CAD build for the part. Positions are in the model's coordinates, mm. A direction names the side the tool comes from. Round coordinates to 2 decimals unless told otherwise and drop trailing zeros. Order: outer loops, then holes, each group sorted by start corner. A loop starts at its lowest first (then second) coordinate and runs counter-clockwise, first axis right, second up. Notation, with made-up numbers: M 34,11 L 55,11 A35 cw 55,44 Z; hole C 60,85 d3. An arc over 180 degrees is marked long. Answer as a JSON object with one key per item and string values.
```python
from build123d import *

# Parameters (mm, degrees)
EXTRUDE_1_DEPTH     = 25
SKETCH_2_R          = 1.7
CUT_EXTRUDE_1_DEPTH = 25
CUT_EXTRUDE_START   = -7.5
SKETCH_3_R          = 2.75
CUT_EXTRUDE_2_DEPTH = 10


with BuildPart() as part:
    # 草图1 → 凸台-拉伸1 (new body)
    with BuildSketch(Plane.XY):
        with BuildLine():
            Line((0, -2.75), (-15.2, -2.75))
            Line((-15.2, -2.75), (-15.2, -1.75))
            Line((-15.2, -1.75), (-2.121320344, -1.75))
            ThreePointArc((-2.121320344, -1.75), (1.17260394, 2.487468593), (0, -2.75))
        make_face()
    extrude(amount=EXTRUDE_1_DEPTH)

    # 草图2 → 切除-拉伸1 (cut)
    with BuildSketch(Plane(origin=(0, -1.75, 0), x_dir=(1, 0, 0), z_dir=(0, 1, 0))):
        with Locations((-10.4, -5.5)):
            Circle(SKETCH_2_R)
        with Locations((-10.4, -19.5)):
            Circle(SKETCH_2_R)
    extrude(amount=-CUT_EXTRUDE_1_DEPTH, mode=Mode.SUBTRACT)

    # 草图3 → 切除-拉伸2 (cut)
    with BuildSketch(Plane(origin=(0, 0, 0), x_dir=(-1, 0, 0), z_dir=(0, 0, -1)).offset(CUT_EXTRUDE_START)):
        Circle(SKETCH_3_R)
    extrude(amount=-CUT_EXTRUDE_2_DEPTH, mode=Mode.SUBTRACT)


solid = part.part
```
Item 1: Drop a flat-ended pin along its axis: pin 1 Ø4 at (x, z) = (-10.4, 5.5) entering from +Y. Give the stop position or say it passes through.
Worked answers:
{"pin 1": "stops at y = -1.75"}
Item 2: Two-plate mould, pull along Z, no slides. Class faces 1 (the flat face through (-2, -1, 0)), 2 (the flat face through (-7, -2.75, 12)), 3 (the cylindrical face through (-8.78, -2.24, 18.99)): released by +Z, released by -Z, zero draft, split by the parting line, or undercut.
Worked answers:
{"face 1": "released by -Z", "face 2": "zero draft", "face 3": "undercut"}
Item 3: Saw through at B-B on z = 19.5. List the corners of the cut face in (x, y).
Worked answers:
{"outline": "M -15.2,-2.75 L -12.1,-2.75 L -12.1,-1.75 L -15.2,-1.75 Z; M -8.7,-2.75 L 0,-2.75 A2.75 ccw long -2.12,-1.75 L -8.7,-1.75 Z"}
Item 4: Wall check: line 1 along Z through (x, y) = (-10.4, -2.15); line 2 along Z through (x, y) = (-9, -2.3); line 3 along Y through (x, z) = (-3.75, 19). Give the ranges that are in metal, low to high. Write a range as [from, to].
Worked answers:
{"line 1": "z = [0, 3.8], [7.2, 17.8], [21.2, 25]", "line 2": "z = [0, 4.54], [6.46, 18.54], [20.46, 25]", "line 3": "y = [-2.75, -1.75]"}
Item 5: Saw through at C-C on y = 0.4. List the corners of the cut face in (x, z).
Worked answers:
{"outline": "M -2.72,0 L 2.72,0 L 2.72,7.5 L -2.72,7.5 Z; M -2.72,17.5 L 2.72,17.5 L 2.72,25 L -2.72,25 Z"}
Item 6: 3-axis set-ups, long thin cutter, end or side, ignore diameter. For faces 4 (the flat face through (0, 0, 7.5)), 5 (the flat face through (-15.2, -2, 12)): which of +Z, -Z, +X, -X, +Y, -Y reach the whole face in a straight line?
Worked answers:
{"face 4": "+X, +Y", "face 5": "+Z, -Z, -X, +Y, -Y"}
Item 7: Saw through at D-D on z = 1.5. List the corners of the cut face in (x, y).
Worked answers:
{"outline": "M -15.2,-2.75 L 0,-2.75 A2.75 ccw long -2.12,-1.75 L -15.2,-1.75 Z"}
Item 8: Saw through at A-A on x = -10.4. List the corners of the cut face in (y, z).
Worked answers:
{"outline": "M -2.75,0 L -1.75,0 L -1.75,3.8 L -2.75,3.8 Z; M -2.75,7.2 L -1.75,7.2 L -1.75,17.8 L -2.75,17.8 Z; M -2.75,21.2 L -1.75,21.2 L -1.75,25 L -2.75,25 Z"}
